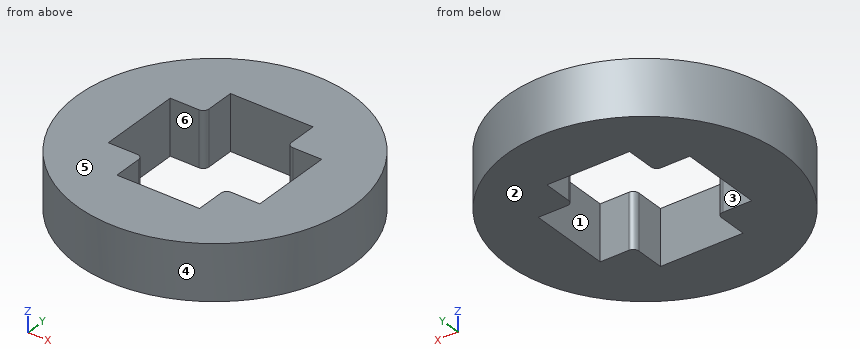
from build123d import *

# Parameters (mm, degrees)
SKETCH1_R           = 5
BOSS_EXTRUDE2_DEPTH = 2
FILLET2_R           = 0.2


with BuildPart() as part:
    # Sketch1 → Boss-Extrude2 (new body)
    with BuildSketch(Plane.XY):
        Circle(SKETCH1_R)
        Polygon((-2.75, -1.5), (-2.75, 1.5), (-1.5, 1.5), (-1.5, 2.75), (1.5, 2.75), (1.5, 1.5), (2.75, 1.5), (2.75, -1.5), (1.5, -1.5), (1.5, -2.75), (-1.5, -2.75), (-1.5, -1.5), align=None, mode=Mode.SUBTRACT)
    extrude(amount=BOSS_EXTRUDE2_DEPTH)

    # Fillet2
    fillet2_edges = [part.edges().sort_by_distance(p)[0] for p in [
        (-1.5, 1.5, 1),
        (-1.5, -1.5, 1),
        (1.5, -1.5, 1),
        (1.5, 1.5, 1),
    ]]
    fillet(fillet2_edges, radius=FILLET2_R)


solid = part.part
Read the model definition and answer for the solid it produces. Units are mm, in the model's axes. Face numbers are marked on the shaded views. A direction names the side the tool comes from. Coordinates: 2 decimals unless noted, no trailing zeros. Order: outer loops, then holes, each group sorted by start corner. A loop starts at its lowest first (then second) coordinate and runs counter-clockwise, first axis right, second up. Notation, with made-up numbers: M -21.75,18.25 L 12.25,18.25 A23 cw 12.25,28.25 Z; hole C 2.5,-23.75 d7. An arc over 180 degrees is marked long. Put each result on its own line as item: value. Start each with the question number.
Item 1: Given pin 1 Ø0.8 at (x, z) = (2, 1) entering from +Y; pin 2 Ø0.6 at (y, z) = (-0.5, 1) entering from -X; pin 3 Ø0.8 at (y, z) = (-2, 1) entering from +X; pin 4 Ø6 at (x, y) = (3, -3.5) entering from -Z, each flat-ended and moving along its own axis, determine where each tip first touches the part or whether it passes through.
Item 2: For the marked faces 5 and 6, determine the directions among +Z, -Z, +X, -X, +Y, -Y from which every point of the face is accessible in a straight line to the end or side of a thin tool.
Item 3: The mould has two halves that part along Y. Classify the marked faces 1, 2, 3 and 4: +Y half, -Y half, draft (parallel to the pull), parting line (faces both ways), or undercut.
Item 4: Section B-B, the plane z = 1.05 is taken. Determine the outline of the cut face in (x, y).
Item 5: Section D-D, the plane x = -4 is taken. Determine the outline of the cut face in (y, z), plus the area to 3 significant figures.
Item 6: Section A-A, the plane x = 0 is taken. Determine the outline of the cut face in (y, z), plus the area to 3 significant figures.
Item 7: Consider probe 1 along X at (y, z) = (-1.25, 1.85); probe 2 along Y at (x, z) = (1, 1.85); probe 3 along X at (y, z) = (2.25, 1.45). Determine where each line is inside the solid, lowest interval first. Write a range as [from, to].
Computed:
1. pin 1: stops at y = 4.74
1. pin 2: stops at x = -5
1. pin 3: stops at x = 4.74
1. pin 4: stops at z = 0
2. face 5: +Z, +X, -X, +Y, -Y
2. face 6: +Z, -Z
3. face 1: undercut
3. face 2: draft
3. face 3: undercut
3. face 4: parting line
4. outline: C 0,0 d10; hole M -2.75,-1.5 L -1.7,-1.5 A0.2 cw -1.5,-1.7 L -1.5,-2.75 L 1.5,-2.75 L 1.5,-1.7 A0.2 cw 1.7,-1.5 L 2.75,-1.5 L 2.75,1.5 L 1.7,1.5 A0.2 cw 1.5,1.7 L 1.5,2.75 L -1.5,2.75 L -1.5,1.7 A0.2 cw -1.7,1.5 L -2.75,1.5 Z
5. outline: M -3,0 L 3,0 L 3,2 L -3,2 Z
5. area: 12.0 mm2
6. outline: M -5,0 L -2.75,0 L -2.75,2 L -5,2 Z; M 2.75,0 L 5,0 L 5,2 L 2.75,2 Z
6. area: 9.00 mm2
7. probe 1: x = [-4.84, -2.75], [2.75, 4.84]
7. probe 2: y = [-4.9, -2.75], [2.75, 4.9]
7. probe 3: x = [-4.47, -1.5], [1.5, 4.47]
